from build123d import *

# Parameters (mm, degrees)
CORTE_EXTRUS_O1_DEPTH      = 74.865587387
CORTE_EXTRUS_O1_DEPTH_BACK = 74.865587387
ESBO_O2_R                  = 4.5
ESBO_O2_R_2                = 2
ESBO_O2_R_3                = 3.5


with BuildPart() as part:
    # Esboço1 → Revolução1 (revolve)
    with BuildSketch(Plane(origin=(0, 0, 0), x_dir=(0, 0, -1), z_dir=(1, 0, 0))):
        with BuildLine():
            Line((-12, 0), (-26, 0))
            ThreePointArc((-26, 0), (-29.327269348, 1.267805111), (-30.967207061, 4.428288525))
            Line((-30.967207061, 4.428288525), (-31.506558588, 9.114342295))
            ThreePointArc((-31.506558588, 9.114342295), (-31.83454613, 9.746438978), (-32.5, 10))
            Line((-32.5, 10), (-51.75, 10))
            Line((-51.75, 10), (-51.75, 12.5))
            Line((-51.75, 12.5), (-32.5, 12.5))
            ThreePointArc((-32.5, 12.5), (-30.170911456, 11.612536422), (-29.022955057, 9.400198032))
            Line((-29.022955057, 9.400198032), (-28.483603531, 4.714144263))
            ThreePointArc((-28.483603531, 4.714144263), (-27.663634674, 3.133902556), (-26, 2.5))
            Line((-26, 2.5), (-12, 2.5))
            Line((-12, 2.5), (-12, 0))
        make_face()
    revolve(axis=Axis((0, 0, 0), (0, -1, 0)))

    # Esboço2 → Corte-extrusão1 (cut, two sides: drawn at the far end of the back side and taken through both)
    with BuildSketch(Plane(origin=(0, 2.5, 0), x_dir=(1, 0, 0), z_dir=(0, 1, 0)).offset(-CORTE_EXTRUS_O1_DEPTH_BACK)):
        with Locations(Location((0, 39.5, 0), (0, 0, 270))):
            Circle(ESBO_O2_R)
        with Locations(Location((-20.931810937, 33.497899798, 0), (0, 0, 270))):
            Circle(ESBO_O2_R_2)
        with Locations(Location((19.125, 33.125471695, 0), (0, 0, 270))):
            Circle(ESBO_O2_R_3)
        with Locations(Location((19.125, -33.125471695, 0), (0, 0, 270))):
            Circle(ESBO_O2_R_3)
        with Locations(Location((34.208003449, -19.75, 0), (0, 0, 270))):
            Circle(ESBO_O2_R)
        with Locations(Location((39.475937667, 1.37853012, 0), (0, 0, 270))):
            Circle(ESBO_O2_R_2)
        with Locations(Location((-38.25, 0, 0), (0, 0, 270))):
            Circle(ESBO_O2_R_3)
        with Locations(Location((-34.208003449, -19.75, 0), (0, 0, 270))):
            Circle(ESBO_O2_R)
        with Locations(Location((-18.54412673, -34.876429918, 0), (0, 0, 270))):
            Circle(ESBO_O2_R_2)
        with BuildLine():
            Line((-7.211102551, 12), (7.211102551, 12))
            ThreePointArc((7.211102551, 12), (14, 0), (7.211102551, -12))
            Line((7.211102551, -12), (-7.211102551, -12))
            ThreePointArc((-7.211102551, -12), (-14, 0), (-7.211102551, 12))
        make_face()
    extrude(amount=CORTE_EXTRUS_O1_DEPTH + CORTE_EXTRUS_O1_DEPTH_BACK, mode=Mode.SUBTRACT)


solid = part.part
The model under review builds one solid part; all positions refer to its coordinate system, in mm. A direction names the side the tool comes from. Coordinates: 2 decimals unless noted, no trailing zeros. Loops run counter-clockwise (first coordinate to the right, second up) from the corner with the lowest first, then second, coordinate; pieces in that order, holes last. Notation, with made-up numbers: M 7,46.25 L 55,46.25 A21 ccw 55,79.25 Z; hole C -34.5,-20 d4. An arc over 180 degrees is marked long. Put each result on its own line as item: value. Start each with the question number.
Q1. Add section C-C (y = 6). Write out the cut boundary in (x, z), and give its area (3 significant figures).
Q2. Add section B-B (z = -39.5). Write out the cut boundary in (x, y).
Q3. For faces 4 (the flat face through (0, 1, -12)), 5 (the flat face through (34, 12.5, -1)), 6 (the flat face through (11, 2.5, 11)), list the 3-axis set-ups (+Z, -Z, +X, -X, +Y, -Y) from which the entire face can be reached by the end or side of a thin tool; tool diameter is ignored.
Q4. Clearance check with flat-ended pins moving along their axes: pin 1 (1 mm diameter, centred on x = 5, y = 11, fed in from -Z); pin 2 (2 mm diameter, centred on x = -3, y = 1, fed in from +Z); pin 3 (3 mm diameter, centred on x = -2, z = 29, fed in from -Y). State where each tip first meets the part, or that it passes through.
Q5. The part is to be moulded in two halves that separate along X. For faces 1 (the conical face through (30.264, 4.721, -6.72)), 2 (the flat face through (-1, 10, -34)), 3 (the cylindrical face through (1.352, 11.233, -35.208)), say which applies: +X half, -X half, draft (parallel to the pull), parting line (faces both ways), or undercut.
Q6. Add section D-D (z = 23). Count the separate pieces of the cut face and the enclosed holes in it, and give its area (3 significant figures).
Q7. Wall thickness on line 1 (Z direction, x = -38.25, y = 11.7); line 2 (Z direction, x = -2, y = 11); line 3 (X direction, y = 11.05, z = 0): over which ranges is each line inside the solid? List them lowest first.
Q8. Add section A-A (x = 0). Write out the cut boundary in (y, z).
Answers:
1. outline: C 0,0 d62.3; hole C 0,0 d57.26
1. area: 473 mm^2
2. outline: M -33.43,10 L -4.5,10 L -4.5,12.5 L -33.43,12.5 Z; M 4.5,10 L 33.43,10 L 33.43,12.5 L 4.5,12.5 Z
3. face 4: +Y, -Y
3. face 5: +Z, -Z, +X, -X, +Y
3. face 6: +Y
4. pin 1: stops at z = -51.55
4. pin 2: stops at z = 29.86
4. pin 3: stops at y = 0.25
5. face 1: parting line
5. face 2: draft
5. face 3: undercut
6. separate pieces: 3
6. enclosed holes: 0
6. area: 255 mm^2
7. line 1: z = -34.86 to -3.5, 3.5 to 17.77, 21.73 to 34.86
7. line 2: z = -51.71 to -43.53, -35.47 to -29.56, 29.56 to 51.71
7. line 3: x = -51.75 to -41.75, -34.75 to -29.66, 29.66 to 38.03, 40.92 to 51.75
8. outline: M 0,-26 A5 ccw 4.43,-30.97 L 9.11,-31.51 A1 cw 10,-32.5 L 10,-35 L 12.5,-35 L 12.5,-32.5 A3.5 ccw 9.4,-29.02 L 4.71,-28.48 A2.5 cw 2.5,-26 L 2.5,-12 L 0,-12 Z; M 0,12 L 2.5,12 L 2.5,26 A2.5 cw 4.71,28.48 L 9.4,29.02 A3.5 ccw 12.5,32.5 L 12.5,51.75 L 10,51.75 L 10,32.5 A1 cw 9.11,31.51 L 4.43,30.97 A5 ccw 0,26 Z; M 10,-51.75 L 12.5,-51.75 L 12.5,-44 L 10,-44 Z
